Autodesk Fusion 360 part; units mm, degrees
sketch "スケッチ1" plane through (0, 0, 0) normal (0, 0, 1) x (1, 0, 0)
  line L0 (2.5, 186) -> (-92.5, 186)
  line L1 (-92.5, 186) -> (-92.5, -186)
  line L2 (-92.5, -186) -> (2.5, -186)
  line L3 (92.5, -150) -> (92.5, 180)
  line L4 (89.5161, 180) -> (-92.5, -186) construction
  line L5 (-92.5, 186) -> (77.5673, -155.9731) construction
  line L6 (2.5, 186) -> (2.5, 180)
  line L7 (2.5, 180) -> (92.5, 180)
  line L8 (-92.5, -186) -> (2.5, -186) construction
  line L9 (2.5, -186) -> (92.5, -150)
  dimension "d2" = 372
  dimension "d5" = 95
extrude "押し出し1" add sketch "スケッチ1" along normal blind 9
chamfer "面取り1" distance 30 angle 45 2 edges at (-92.5, -186, 4.5) (-92.5, 186, 4.5)
sketch "スケッチ2" plane through (0, 0, 9) normal (0, 0, 1) x (-1, 0, 0)
  line L0 (62.5, -186) -> (92.5, -156)
  line L1 (92.5, -156) -> (92.5, 156)
  line L2 (92.5, 156) -> (62.5, 186)
  line L3 (62.5, 186) -> (-2.5, 186)
  line L4 (-2.5, 186) -> (-92.5, 150)
  line L5 (-92.5, 150) -> (-92.5, -180)
  line L6 (-92.5, -180) -> (-2.5, -180)
  line L7 (-2.5, -180) -> (-2.5, -186)
  line L8 (-2.5, -186) -> (62.5, -186)
  line L9 (-92.5, -180) -> (-52.5, -180) construction
  line L10 (-52.5, -180) -> (-52.5, -130) construction
  line L11 (-52.5, -130) -> (-92.5, -130) construction
  line L12 (-92.5, -130) -> (-92.5, -180) construction
  line L13 (-52.5, -130) -> (-52.5, -60) construction
  line L14 (-52.5, -60) -> (-52.5, 10) construction
  line L15 (-52.5, 10) -> (-52.5, 80) construction
  point P0 (-52.5, -130)
  point P1 (-52.5, -60)
  point P2 (-52.5, 10)
  point P3 (-52.5, 80)
  dimension "d10" = 40
  dimension "d11" = 50
  dimension "d12" = 70
  dimension "d13" = 70
  dimension "d14" = 70
hole "穴1" at (52.5, 130, 9) at (52.5, 60, 9) at (52.5, -10, 9) at (52.5, -80, 9) direction (0, 0, -1) diameter 22 end through all
equation "d5 = 30 mm + 65 mm"
CAD build for the part. Positions are in the model's coordinates, mm. A direction names the side the tool comes from. Round coordinates to 2 decimals unless told otherwise and drop trailing zeros. Write each loop counter-clockwise with the first axis right and the second up, starting at its lowest first coordinate (ties: lowest second). Pieces come first, ordered by that corner, then holes. Notation, with made-up numbers: (8.25, -32.75) - (22.25, -32.75) arc R28 cw to (22.25, 6.25) - close; hole circle Ø3 at (87.5, 18.25). An arc over 180 degrees is marked (long way). Write item = value, one per line. Start each with the question number.
Q1. Probe L1, parallel to X at y = -80, z = 6; L2, parallel to Y at x = 52.5, z = 3; L3, parallel to Y at x = 53.5, z = 3.75. List the from-to ranges inside material, lowest first. Write a range as from..to.
Q2. Band-saw the part on B-B (y = -80). Give the cut face in (x, z).
Q3. Mould opens along X. For faces 1 (the cylindrical face through (45.07, -71.89, 4.44)), 2 (the cylindrical face through (52.02, 140.99, 4.44)), 3 (the flat face through (92.5, 13, 4)), 4 (the flat face through (-30, 186, 4)) say: pulls with the +X half, pulls with the -X half, needs draft (parallel to the pull), parting line crosses it, or undercut.
Q4. Band-saw the part on D-D (y = 56.5). Give the cut face in (x, z), then the cut area to 3 significant figures.
Q5. Band-saw the part on A-A (x = 52.5). Give the cut face in (y, z), then the cut area to 3 significant figures.
Q6. Band-saw the part on C-C (z = 6). Give the cut face in (x, y), then the cut area to 3 significant figures.
Q7. Drop a flat-ended pin along its axis: pin 1 (1.5 mm diameter, centred on x = 71, z = 3, fed in from +Y). Give the stop position or say it passes through.
Q8. Which spindle directions (+Z, -Z, +X, -X, +Y, -Y) get a long thin tool onto all of the face, cutting with end or side? Do faces 5 (the flat face through (47, 180, 4)), 6 (the flat face through (46.87, -168.25, 4.44)). Say none if no direction does.
Answers below:
q1.L1 = -92.5..41.5, 63.5..92.5
q1.L2 = -166..-91, -69..-21, 1..49, 71..119, 141..180
q1.L3 = -165.6..-90.95, -69.05..-20.95, 0.95..49.05, 70.95..119.05, 140.95..180
q2.outline = (-92.5, 0) - (41.5, 0) - (41.5, 9) - (-92.5, 9) - close; (63.5, 0) - (92.5, 0) - (92.5, 9) - (63.5, 9) - close
q3.face_1 = undercut
q3.face_2 = undercut
q3.face_3 = pulls with the +X half
q3.face_4 = needs draft
q4.outline = (-92.5, 0) - (42.07, 0) - (42.07, 9) - (-92.5, 9) - close; (62.93, 0) - (92.5, 0) - (92.5, 9) - (62.93, 9) - close
q4.area = 1,480 mm2
q5.outline = (-166, 0) - (-91, 0) - (-91, 9) - (-166, 9) - close; (-69, 0) - (-21, 0) - (-21, 9) - (-69, 9) - close; (1, 0) - (49, 0) - (49, 9) - (1, 9) - close; (71, 0) - (119, 0) - (119, 9) - (71, 9) - close; (141, 0) - (180, 0) - (180, 9) - (141, 9) - close
q5.area = 2,320 mm2
q6.outline = (-92.5, -156) - (-62.5, -186) - (2.5, -186) - (92.5, -150) - (92.5, 180) - (2.5, 180) - (2.5, 186) - (-62.5, 186) - (-92.5, 156) - close; hole circle Ø22 at (52.5, -80); hole circle Ø22 at (52.5, -10); hole circle Ø22 at (52.5, 60); hole circle Ø22 at (52.5, 130)
q6.area = 64,200 mm2
q7.pin_1 = 180
q8.face_5 = +Z, -Z, +X, +Y
q8.face_6 = +Z, -Z, +X, -Y
